Work out the finished part from the listing and answer in its coordinate system (mm). Coordinates: 2 decimals unless noted, no trailing zeros. Order: outer loops, then holes, each group sorted by start corner. A loop starts at its lowest first (then second) coordinate and runs counter-clockwise, first axis right, second up. Notation, with made-up numbers: M 39,49.5 L 65,49.5 A7 cw 65,62.5 Z; hole C 58,-38.75 d2. An arc over 180 degrees is marked long. Use a Markdown table: item, result.
Autodesk Inventor part; units mm, degrees
ref_plane "YZ Plane" through (0, 0, 0) normal (1, 0, 0) x (0, 1, 0)
ref_plane "XZ Plane" through (0, 0, 0) normal (0, 1, 0) x (-1, 0, 0)
ref_plane "XY Plane" through (0, 0, 0) normal (0, 0, 1) x (1, 0, 0)
sketch "Sketch1" plane through (0, 0, 0) normal (0, 0, 1) x (1, 0, 0)
  line L0 (0, 0) -> (1.27, 0)
  line L1 (3.175, 12.7) -> (3.175, 90.4875)
  line L2 (3.175, 90.4875) -> (0, 90.4875)
  line L3 (0, 90.4875) -> (0, 0)
  line L4 (1.27, 0) -> (3.175, 12.7)
  dimension "d0" = 3.175
  dimension "d1" = 77.7875
  dimension "d2" = 1.27
  dimension "d3" = 12.7
revolve "Revolution1" add sketch "Sketch1" angle 360 about axis through (0, 90.4875, 0) along (0, -1, 0)
shell "Shell1" thickness 0.635 removed faces 2 at (-0.5202, 90.4875, -0.7796) at (-0.1274, 0, 0.3526)
fillet "Fillet1" radius 3.175 1 edges at (-3.175, 12.7, 0)
properties part number "Pipette" material "Glass"
1. Section A-A on y = 72 is taken. Determine the outline of the cut face in (x, z) (3 decimals), then the cut area to 3 significant figures.
Answers below:
| item | result |
|---|---|
| outline | C 0,0 d6.35; hole C 0,0 d5.08 |
| area | 11.4 mm² |
2. Flat-ended cylindrical pins translate along their axes: P1, Ø1, axis at x = -1.5, y = 26, coming from the -Z side; P2, Ø2, axis at x = 2, y = 73, coming from the +Z side; P3, Ø3, axis at x = -2, y = 71.5, coming from the -Z side; P4, Ø2, axis at x = 1, y = 43.5, coming from the -Z side (3 decimals). Find the tip coordinate at first contact, or state that the pin passes through.
Answers below:
| item | result |
|---|---|
| P1 | z = -3.01 |
| P2 | z = 3.01 |
| P3 | z = -3.14 |
| P4 | z = -3.175 |
3. Find the intervals of material crossed by probe 1 along X at (y, z) = (34.5, 0) (3 decimals); probe 2 along X at (y, z) = (45, 0.75), in increasing order.
Answers below:
| item | result |
|---|---|
| probe 1 | -3.175 to -2.54, 2.54 to 3.175 |
| probe 2 | -3.09 to -2.43, 2.43 to 3.09 |
4. For a pull along Z with two mould halves and no side action, classify faces 1 (the face through (-1, 0, 0)), 2 (the face through (-0.33, 52.16, -2.52)), 3 (the face through (-0.29, 6.32, -2.2)) as +Z half, -Z half, draft (parallel to the pull), parting line (faces both ways), or undercut.
Answers below:
| item | result |
|---|---|
| face 1 | draft |
| face 2 | undercut |
| face 3 | parting line |
